from build123d import *

# Parameters (mm, degrees)
F1_DEPTH  = 19
F2_R      = 11.25
F3_DEPTH  = 0.8
F4_R      = 8
F5_DEPTH  = 17
F7_DEPTH  = 25
F9_DEPTH  = 25
F11_DEPTH = 30.05913
F14_R     = 8
F15_DEPTH = 25


with BuildPart() as f1:
    # F0 (on Top) → F1 (new body)
    with BuildSketch(Plane.XY):
        Polygon((0, -12), (0, 0), (0, 12), (-6.928203, 12), (-13.856406, 0), (-6.928203, -12), align=None)
        Polygon((0, 12), (0, 0), (0, -12), (6.928203, -12), (13.856406, 0), (6.928203, 12), align=None)
    extrude(amount=F1_DEPTH)

    # F2 (on face) → F3 (join)
    with BuildSketch(Plane(origin=(0, 0, 0), x_dir=(1, 0, 0), z_dir=(0, 0, -1))):
        Circle(F2_R)
    extrude(amount=F3_DEPTH)

    # F4 (on face) → F5 (cut)
    with BuildSketch(Plane.XY.offset(19)):
        Circle(F4_R)
    extrude(amount=-F5_DEPTH, mode=Mode.SUBTRACT)

    # F6 (on face) → F7 (cut)
    with BuildSketch(Plane(origin=(10.392305, -6, 0), x_dir=(0.5, 0.866025, 0), z_dir=(0.866025, -0.5, 0))):
        with BuildLine():
            Line((0, 19), (-2.25, 19))
            Line((-2.25, 19), (-2.25, 15.25))
            ThreePointArc((-2.25, 15.25), (0, 13), (2.25, 15.25))
            Line((2.25, 15.25), (2.25, 19))
            Line((2.25, 19), (0, 19))
        make_face()
    extrude(amount=-F7_DEPTH, mode=Mode.SUBTRACT)

    # F8 (on face) → F9 (cut)
    with BuildSketch(Plane(origin=(-10.392305, -6, 0), x_dir=(0.5, -0.866025, 0), z_dir=(-0.866025, -0.5, 0))):
        with BuildLine():
            Line((2.25, 19), (0, 19))
            Line((0, 19), (-2.25, 19))
            Line((-2.25, 19), (-2.25, 15.25))
            ThreePointArc((-2.25, 15.25), (0, 13), (2.25, 15.25))
            Line((2.25, 15.25), (2.25, 19))
        make_face()
    extrude(amount=-F9_DEPTH, mode=Mode.SUBTRACT)

    # F10 (on face) → F11 (cut)
    with BuildSketch(Plane.XZ.offset(12)):
        with BuildLine():
            ThreePointArc((-2.25, 15.25), (0, 13), (2.25, 15.25))
            Line((2.25, 15.25), (2.25, 19))
            Line((2.25, 19), (0, 19))
            Line((0, 19), (-2.25, 19))
            Line((-2.25, 19), (-2.25, 15.25))
        make_face()
    extrude(amount=-F11_DEPTH, mode=Mode.SUBTRACT)

    # F12 (on Front) → F13 (revolve, cut)
    with BuildSketch(Plane.XZ):
        with BuildLine():
            ThreePointArc((8.079038, 23.642426), (13.284742, 17.664152), (16.167056, 10.279615))
            Line((16.167056, 10.279615), (18.863061, 27.862262))
            Line((18.863061, 27.862262), (8.079038, 23.642426))
        make_face()
    revolve(axis=Axis((0, 0, -20.240964), (0, 0, -1)), mode=Mode.SUBTRACT)

    # F14 (on face) → F15 (cut)
    with BuildSketch(Plane(origin=(0, 0, -0.8), x_dir=(1, 0, 0), z_dir=(0, 0, -1))):
        Circle(F14_R)
    extrude(amount=-F15_DEPTH, mode=Mode.SUBTRACT)


solid = f1.part
The listing builds one solid part. Answer for the finished solid, in the listing's coordinates (mm). A direction names the side the tool comes from. Give positions to 0.01 mm unless a question says otherwise; leave off trailing zeros. Write each loop counter-clockwise with the first axis right and the second up, starting at its lowest first coordinate (ties: lowest second). Pieces come first, ordered by that corner, then holes. Notation, with made-up numbers: (23.5, -22) - (30.5, -22) arc R21 ccw to (30.5, -12) - close; hole circle Ø1 at (70, -10). An arc over 180 degrees is marked (long way). One line per question, with ' | ' between items. Start each with the question number.
1. Section B-B, the plane x = 0 is taken. Determine the outline of the cut face in (y, z), then the cut area to 3 significant figures.
2. For faces 1 (the face through (7.42, -6.88, 17.15)), 2 (the face through (10.2, -5.3, 0)), 3 (the face through (9.619, 2.956, 17.099)), determine the directions among +Z, -Z, +X, -X, +Y, -Y from which every point of the face is accessible in a straight line to the end or side of a thin tool.
3. Determine the mould class of faces 4 (the face through (3.69, -7.1, 7.04)), 5 (the face through (-10.44, -5.92, 9.37)), 6 (the face through (2.25, 10, 17)) for opening direction Y: +Y half, -Y half, draft (parallel to the pull), parting line (faces both ways), or undercut.
4. Straight lines are drawn through the part: line 1 (Y direction, x = 0, z = 12.25); line 2 (Z direction, x = 0, y = -9); line 3 (Z direction, x = 12, y = 2.5). For each, find the intervals that lie inside material, in ascending order.
5. Section C-C, the plane z = 14.75 is taken. Count the separate pieces of the cut face and the enclosed holes in it, then the cut area to 3 significant figures.
6. Section A-A, the plane z = 4 is taken. Determine the outline of the cut face in (x, y), then the cut area to 3 significant figures.
7. Given P1, Ø4, axis at x = 8, z = 8, coming from the +Y side; P2, Ø4, axis at y = 9.5, z = 18, coming from the +X side; P3, Ø3, axis at x = -11, z = 6, coming from the +Y side; P4, Ø3, axis at x = 10.5, z = 7.5, coming from the +Y side, each flat-ended and moving along its own axis, determine where each tip first touches the part or whether it passes through.
Result:
1) outline: (-12, 0) - (-11.25, 0) - (-11.25, -0.8) - (-8, -0.8) - (-8, 13) - (-12, 13) - close; (8, -0.8) - (11.25, -0.8) - (11.25, 0) - (12, 0) - (12, 13) - (8, 13) - close | area: 109 mm2
2) face 1: +Z, +X | face 2: -Z | face 3: +Z
3) face 4: undercut | face 5: -Y half | face 6: draft
4) line 1: y = -12 to -8, 8 to 12 | line 2: z = -0.8 to 13 | line 3: z = 0 to 19
5) separate pieces: 6 | enclosed holes: 0 | area: 190 mm2
6) outline: (-13.86, 0) - (-6.93, -12) - (6.93, -12) - (13.86, 0) - (6.93, 12) - (-6.93, 12) - close; hole circle Ø16 at (0, 0) | area: 298 mm2
7) P1: stops at y = 12 | P2: stops at x = 9.27 | P3: stops at y = 7.55 | P4: stops at y = 8.41
